```python
from build123d import *

# Parameters (mm, degrees)
F0_W      = 25.4
F0_H      = 25.4
F1_DEPTH  = 25.4
F2_R      = 3.302351
F3_DEPTH  = 0.5
F4_R      = 3.247176
F4_R_2    = 2.961893
F5_DEPTH  = 0.5
F6_R      = 3.005725
F6_R_2    = 2.980897
F6_R_3    = 3.094584
F7_DEPTH  = 0.5
F8_R      = 3.319933
F8_R_2    = 3.427054
F8_R_3    = 3.00862
F8_R_4    = 3.51795
F9_DEPTH  = 0.5
F10_R     = 3.021029
F10_R_2   = 3.181176
F10_R_3   = 2.727784
F10_R_4   = 3.452089
F10_R_5   = 2.749013
F11_DEPTH = 0.5
F12_R     = 3.134358
F12_R_2   = 3.167686
F12_R_3   = 3.143619
F12_R_4   = 3.049756
F12_R_5   = 3.227009
F12_R_6   = 3.40973
F13_DEPTH = 0.5


with BuildPart() as f1:
    # F0 (on Top) → F1 (new body)
    with BuildSketch(Plane.XY):
        Rectangle(F0_W, F0_H)
    extrude(amount=F1_DEPTH)

    # F2 (on face) → F3 (join)
    with BuildSketch(Plane(origin=(0, 12.7, 0), x_dir=(-1, 0, 0), z_dir=(0, 1, 0))):
        with Locations((0, 12.774332)):
            Circle(F2_R)
    extrude(amount=F3_DEPTH)

    # F4 (on face) → F5 (join)
    with BuildSketch(Plane(origin=(0, 0, 0), x_dir=(1, 0, 0), z_dir=(0, 0, -1))):
        with Locations((0, -5.861166)):
            Circle(F4_R)
        with Locations((0, 6.762884)):
            Circle(F4_R_2)
    extrude(amount=F5_DEPTH)

    # F6 (on face) → F7 (join)
    with BuildSketch(Plane.XY.offset(25.4)):
        with Locations((8.356908, -8.566318)):
            Circle(F6_R)
        Circle(F6_R_2)
        with Locations((-8.475154, 9.468036)):
            Circle(F6_R_3)
    extrude(amount=F7_DEPTH)

    # F8 (on face) → F9 (join)
    with BuildSketch(Plane.XZ.offset(12.7)):
        with Locations((-6.671718, 8.566318)):
            Circle(F8_R)
        with Locations((4.449466, 9.167464)):
            Circle(F8_R_2)
        with Locations((-7.574594, 18.485788)):
            Circle(F8_R_3)
        with Locations((4.449466, 19.689236)):
            Circle(F8_R_4)
    extrude(amount=F9_DEPTH)

    # F10 (on face) → F11 (join)
    with BuildSketch(Plane(origin=(-12.7, 0, 0), x_dir=(0, -1, 0), z_dir=(-1, 0, 0))):
        with Locations((-8.876446, 4.915892)):
            Circle(F10_R)
        with Locations((0, 12.872338)):
            Circle(F10_R_2)
        with Locations((-9.358654, 21.310989)):
            Circle(F10_R_3)
        with Locations((8.724171, 20.82878)):
            Circle(F10_R_4)
        with Locations((8.724171, 5.156996)):
            Circle(F10_R_5)
    extrude(amount=F11_DEPTH)

    # F12 (on face) → F13 (join)
    with BuildSketch(Plane.YZ.offset(12.7)):
        with Locations((-8.394237, 6.362522)):
            Circle(F12_R)
        with Locations((0, 6.362522)):
            Circle(F12_R_2)
        with Locations((8.724171, 6.362522)):
            Circle(F12_R_3)
        with Locations((-9.11755, 17.212216)):
            Circle(F12_R_4)
        with Locations((0, 17.694423)):
            Circle(F12_R_5)
        with Locations((8.724171, 18.658841)):
            Circle(F12_R_6)
    extrude(amount=F13_DEPTH)


solid = f1.part
```
Geometry check sheet. Reference: the model listing, model coordinates, mm. A direction names the side the tool comes from. Round coordinates to 2 decimals unless told otherwise and drop trailing zeros. Order: outer loops, then holes, each group sorted by start corner. A loop starts at its lowest first (then second) coordinate and runs counter-clockwise, first axis right, second up. Notation, with made-up numbers: M 4.5,20.25 L 34.5,20.25 A10 ccw 34.5,26.25 Z; hole C 51,68 d1. An arc over 180 degrees is marked long. Write item = value, one per line.
Q1. Section check D-D (y = -7.5). Enter the section's corners in (x, z).
Answer block:
outline = M -13.2,2.7 L -12.7,2.7 L -12.7,0 L -2.87,0 L -2.87,-0.5 L 2.87,-0.5 L 2.87,0 L 12.7,0 L 12.7,3.36 L 13.2,3.36 L 13.2,9.37 L 12.7,9.37 L 12.7,14.63 L 13.2,14.63 L 13.2,19.8 L 12.7,19.8 L 12.7,25.4 L 11.17,25.4 L 11.17,25.9 L 5.55,25.9 L 5.55,25.4 L -12.7,25.4 L -12.7,24.06 L -13.2,24.06 L -13.2,17.6 L -12.7,17.6 L -12.7,7.62 L -13.2,7.62 Z
Q2. Release check for a two-part mould opening along Z. For faces 6 (the cylindrical face through (-2.37, -1.81, 25.65)), 7 (the cylindrical face through (12.946, -0.412, 9.503)), 8 (the flat face through (0, 0, 0)) record: released by +Z, released by -Z, zero draft, split by the parting line, or undercut.
Answer block:
face_6 = zero draft
face_7 = undercut
face_8 = released by -Z
Q3. Scan lines: line 1 (Z direction, x = -3, y = 6.75); line 2 (Z direction, x = 7, y = -4.5); line 3 (Y direction, x = 2.5, z = 18.5). Record each from-to range of solid material in increasing order.
Answer block:
line_1 = -0.5 to 25.4
line_2 = 0 to 25.4
line_3 = -13.2 to 12.7
Q4. Set-up check for faces 1 (the cylindrical face through (0.72, 12.95, 9.55)), 2 (the cylindrical face through (3.1, 4.9, -0.2)), 3 (the flat face through (0, -12.7, 13)), 4 (the flat face through (-12.7, -3, 10)), 5 (the cylindrical face through (12.95, 11.72, 7.31)): record each of +Z, -Z, +X, -X, +Y, -Y from which the full face is reachable in a straight line by a thin tool's end or side.
Answer block:
face_1 = +Y
face_2 = -Z
face_3 = -Y
face_4 = -X
face_5 = +X
Q5. Section check C-C (z = 3.75). Enter the section's corners in (x, y).
Answer block:
outline = M -13.2,-11.09 L -12.7,-11.09 L -12.7,-12.7 L 12.7,-12.7 L 12.7,-10.13 L 13.2,-10.13 L 13.2,-6.66 L 12.7,-6.66 L 12.7,-1.79 L 13.2,-1.79 L 13.2,1.79 L 12.7,1.79 L 12.7,6.98 L 13.2,6.98 L 13.2,10.47 L 12.7,10.47 L 12.7,12.7 L -12.7,12.7 L -12.7,11.66 L -13.2,11.66 L -13.2,6.09 L -12.7,6.09 L -12.7,-6.36 L -13.2,-6.36 Z
Q6. Depth check by flat-ended pin: pin 1 Ø1.5 at (x, z) = (-2, 10.5) entering from -Y; pin 2 Ø2 at (x, y) = (3, -7.5) entering from +Z; pin 3 Ø8 at (x, y) = (-9.5, 2) entering from -Z. Enter the tip coordinate at first touch or a pass-through.
Answer block:
pin_1 = -12.7
pin_2 = 25.4
pin_3 = 0
Q7. Section check B-B (x = 0). Enter the section's corners in (y, z).
Answer block:
outline = M -12.7,0 L -9.72,0 L -9.72,-0.5 L -3.8,-0.5 L -3.8,0 L 2.61,0 L 2.61,-0.5 L 9.11,-0.5 L 9.11,0 L 12.7,0 L 12.7,9.47 L 13.2,9.47 L 13.2,16.08 L 12.7,16.08 L 12.7,25.4 L 2.98,25.4 L 2.98,25.9 L -2.98,25.9 L -2.98,25.4 L -12.7,25.4 Z
Q8. Section check A-A (y = 0). Enter the section's corners in (x, z).
Answer block:
outline = M -13.2,9.69 L -12.7,9.69 L -12.7,0 L 12.7,0 L 12.7,3.19 L 13.2,3.19 L 13.2,9.53 L 12.7,9.53 L 12.7,14.47 L 13.2,14.47 L 13.2,20.92 L 12.7,20.92 L 12.7,25.4 L 2.98,25.4 L 2.98,25.9 L -2.98,25.9 L -2.98,25.4 L -12.7,25.4 L -12.7,16.05 L -13.2,16.05 Z
